For this review, take the finished solid that the model builds, in its own axes (mm). Round coordinates to 2 decimals unless told otherwise and drop trailing zeros. Write each loop counter-clockwise with the first axis right and the second up, starting at its lowest first coordinate (ties: lowest second). Pieces come first, ordered by that corner, then holes. Notation, with made-up numbers: (45.5, 15) - (89.5, 15) arc R34 cw to (89.5, 48) - close; hole circle Ø3 at (-11, -18.5). An arc over 180 degrees is marked (long way). One line per item, written item: value. Start each with the question number.
Q1. Clearance check with flat-ended pins moving along their axes: pin 1 Ø1.6 at (y, z) = (-16, 23) entering from -X; pin 2 Ø1 at (x, y) = (-7, 16) entering from +Z; pin 3 Ø1.5 at (x, z) = (91.5, 10) entering from +Y; pin 4 Ø2 at (x, y) = (108.5, -47.5) entering from +Z. State where each tip first meets the part, or that it passes through.
Q2. Add section B-B on y = -9. Write out the cut boundary in (x, z), and give its area (3 significant figures).
Q3. Add section C-C on x = 42.75. Write out the cut boundary in (y, z).
Q4. For probe 1 along Y at (x, z) = (94.5, 43.5); probe 2 along Y at (x, z) = (70, 2.35); probe 3 along Z at (x, y) = (17, -19), list the stretches that pass through material, from the lowest coordinate up.
Q5. Add section D-D on x = -28. Write out the cut boundary in (y, z), and give its area (3 significant figures).
Q6. Mouldability with a two-part tool opening along Y and no side actions: class faces 1 (the face through (76, 17, 28)), 2 (the face through (59, 15, 27)), 3 (the face through (46.211, 15.986, 22.346)) as +Y half, -Y half, draft (parallel to the pull), parting line (faces both ways), or undercut.
Q7. Add section A-A on z = 33.5. Write out the cut boundary in (x, y), and give its area (3 significant figures).
```python
from build123d import *

# Parameters (mm, degrees)
SZKIC1_W                    = 260
SZKIC1_H                    = 150
DODANIE_WYCI_GNI_CIE1_DEPTH = 3
SZKIC2_R                    = 2.5
SZKIC2_W                    = 155
SZKIC2_H                    = 30
WYTNIJ_WYCI_GNI_CIE1_DEPTH  = 3
WYTNIJ_WYCI_GNI_CIE3_DEPTH  = 3
SZKIC6_W                    = 155
SZKIC6_H                    = 2
DODANIE_WYCI_GNI_CIE2_DEPTH = 5
SZKIC7_W                    = 77.5
SZKIC7_H                    = 2
DODANIE_WYCI_GNI_CIE3_DEPTH = 48
SZKIC10_W                   = 20
SZKIC10_H                   = 48
DODANIE_WYCI_GNI_CIE5_DEPTH = 2
SZKIC12_R                   = 7.5
WYTNIJ_WYCI_GNI_CIE4_DEPTH  = 40
ZAOKR_GLENIE1_R             = 10


with BuildPart() as part:
    # Szkic1 → Dodanie-wyciągnięcie1 (new body)
    with BuildSketch(Plane.XY):
        Rectangle(SZKIC1_W, SZKIC1_H)
    extrude(amount=DODANIE_WYCI_GNI_CIE1_DEPTH)

    # Szkic2 → Wytnij-wyciągnięcie1 (cut)
    with BuildSketch(Plane.XY.offset(3)):
        with Locations((70, 25)):
            Circle(SZKIC2_R)
        with Locations((70, -25)):
            Circle(SZKIC2_R)
        with Locations((42.5, 0)):
            Rectangle(SZKIC2_W, SZKIC2_H)
    extrude(amount=-WYTNIJ_WYCI_GNI_CIE1_DEPTH, mode=Mode.SUBTRACT)

    # Szkic4 → Wytnij-wyciągnięcie3 (cut)
    with BuildSketch(Plane(origin=(0, 0, 0), x_dir=(-1, 0, 0), z_dir=(0, 0, -1))):
        with BuildLine():
            ThreePointArc((-123.23193039, -39.89969852), (-128.133858368, -36.253613669), (-130, -30.436367925))
            Line((-130, -30.436367925), (-130, -75))
            Line((-130, -75), (130, -75))
            Line((130, -75), (130, 75))
            Line((130, 75), (-130, 75))
            Line((-130, 75), (-130, 33.178745855))
            ThreePointArc((-130, 33.178745855), (-128.050508227, 39.11080429), (-122.962136544, 42.729962902))
            Line((-122.962136544, 42.729962902), (-68.723094228, 59.551217048))
            ThreePointArc((-68.723094228, 59.551217048), (-66.430659203, 59.977549793), (-64.101812385, 59.861401365))
            Line((-64.101812385, 59.861401365), (56.659145299, 39.543804725))
            ThreePointArc((56.659145299, 39.543804725), (62.635163816, 36.140287961), (65, 29.682403361))
            Line((65, 29.682403361), (65, -22.197400037))
            ThreePointArc((65, -22.197400037), (62.841744534, -28.402804348), (57.298591466, -31.929639105))
            Line((57.298591466, -31.929639105), (-60.417650648, -59.732239068))
            ThreePointArc((-60.417650648, -59.732239068), (-63.201894591, -59.988200122), (-65.948172504, -59.463330595))
            Line((-65.948172504, -59.463330595), (-123.23193039, -39.89969852))
        make_face()
    extrude(amount=-WYTNIJ_WYCI_GNI_CIE3_DEPTH, mode=Mode.SUBTRACT)

    # Szkic6 → Dodanie-wyciągnięcie2 (add)
    with BuildSketch(Plane(origin=(0, 0, 0), x_dir=(-1, 0, 0), z_dir=(0, 0, -1))):
        with Locations((-42.5, 16)):
            Rectangle(SZKIC6_W, SZKIC6_H)
        with Locations((-42.5, -16)):
            Rectangle(SZKIC6_W, SZKIC6_H)
    extrude(amount=-DODANIE_WYCI_GNI_CIE2_DEPTH)

    # Szkic7 → Dodanie-wyciągnięcie3 (add)
    with BuildSketch(Plane.XY.offset(5)):
        with Locations((81.25, 16)):
            Rectangle(SZKIC7_W, SZKIC7_H)
    dodanie_wyci_gni_cie3 = extrude(amount=DODANIE_WYCI_GNI_CIE3_DEPTH)

    # Lustro2: Dodanie-wyciągnięcie3 across plane
    add(dodanie_wyci_gni_cie3.mirror(Plane.ZX))

    # Szkic10 → Dodanie-wyciągnięcie5 (add)
    with BuildSketch(Plane.XZ.offset(17)):
        with Locations((32.5, 29)):
            Rectangle(SZKIC10_W, SZKIC10_H)
    dodanie_wyci_gni_cie5 = extrude(amount=-DODANIE_WYCI_GNI_CIE5_DEPTH)

    # Lustro3: Dodanie-wyciągnięcie5 across plane
    add(dodanie_wyci_gni_cie5.mirror(Plane.ZX))

    # Szkic12 → Wytnij-wyciągnięcie4 (cut)
    with BuildSketch(Plane(origin=(0, -17, 0), x_dir=(-1, 0, 0), z_dir=(0, -1, 0))):
        with Locations(Location((-42.75, -29, 0), (0, 0, 180))):
            Circle(SZKIC12_R)
    extrude(amount=-WYTNIJ_WYCI_GNI_CIE4_DEPTH, mode=Mode.SUBTRACT)

    # Zaokrąglenie1
    zaokr_glenie1_edges = [part.edges().sort_by_distance(p)[0] for p in [
        (120, 16, 53),
        (120, -16, 53),
        (22.5, -16, 53),
        (22.5, 16, 53),
    ]]
    fillet(zaokr_glenie1_edges, radius=ZAOKR_GLENIE1_R)


solid = part.part
```
Result set:
1. pin 1: stops at x = 22.5
1. pin 2: stops at z = 5
1. pin 3: stops at y = 17
1. pin 4: passes through
2. outline: (-65, 0) - (-35, 0) - (-35, 3) - (-65, 3) - close; (120, 0) - (130, 0) - (130, 3) - (120, 3) - close
2. area: 120 mm^2
3. outline: (-55.56, 0) - (-15, 0) - (-15, 21.5) - (-17, 21.5) - (-17, 3) - (-55.56, 3) - close; (-17, 36.5) - (-15, 36.5) - (-15, 53) - (-17, 53) - close; (15, 0) - (56.27, 0) - (56.27, 3) - (17, 3) - (17, 21.5) - (15, 21.5) - close; (15, 36.5) - (17, 36.5) - (17, 53) - (15, 53) - close
4. probe 1: y = -17 to -15, 15 to 17
4. probe 2: y = -58.08 to -27.5, -22.5 to -15, 15 to 22.5, 27.5 to 59.16
4. probe 3: z = 0 to 3
5. outline: (-38.85, 0) - (-15, 0) - (-15, 5) - (-17, 5) - (-17, 3) - (-38.85, 3) - close; (15, 0) - (44.37, 0) - (44.37, 3) - (17, 3) - (17, 5) - (15, 5) - close
5. area: 168 mm^2
6. face 1: +Y half
6. face 2: undercut
6. face 3: draft
7. outline: (22.5, -17) - (36.75, -17) - (36.75, -15) - (22.5, -15) - close; (22.5, 15) - (36.75, 15) - (36.75, 17) - (22.5, 17) - close; (48.75, -17) - (120, -17) - (120, -15) - (48.75, -15) - close; (48.75, 15) - (120, 15) - (120, 17) - (48.75, 17) - close
7. area: 342 mm^2
